Source: CAD feature listing. Evaluate the final solid. Frame: model axes, mm. A direction names the side the tool comes from. Give positions to 0.01 mm unless a question says otherwise; leave off trailing zeros. Loops run counter-clockwise (first coordinate to the right, second up) from the corner with the lowest first, then second, coordinate; pieces in that order, holes last. Notation, with made-up numbers: (18.5, 65.25) -> (40.5, 65.25) arc R21 cw to (40.5, 97.25) -> close; hole circle Ø6 at (32.5, 88). An arc over 180 degrees is marked (long way). Return JSON: item names as keys, results as strings. Group by question number.
Autodesk Inventor part; units mm, degrees
ref_plane "Work Plane1" through (0, 108.1, -624) normal (0, 0, 1) x (1, 0, 0)
ref_plane "YZ Plane" through (0, 0, 0) normal (1, 0, 0) x (0, 1, 0)
ref_plane "XZ Plane" through (0, 0, 0) normal (0, 1, 0) x (-1, 0, 0)
sketch "Sketch1" plane through (0, 0, 0) normal (1, 0, 0) x (0, 1, 0)
  line L0 (107.6, 0) -> (-107.6, 0) construction
  line L1 (108.1, 0) -> (108.1, -40)
  line L2 (108.1, -40) -> (112.1, -40)
  line L3 (112.1, -40) -> (112.1, 12.9)
  line L4 (0, 0) -> (0, 125)
  arc A0 (112.1, 12.9) -> (0, 125) centre (0, 12.9) ccw
  line L5 (108.1, 0) -> (0, 0)
  line L6 (98.1, 0) -> (98.1, 12.9)
  arc A1 (98.1, 12.9) -> (0, 111) centre (0, 12.9) ccw
  line L7 (99.6, 0) -> (99.6, -254) construction
  line L8 (107.6, -254) -> (107.6, 0) construction
  dimension "d0" = 125
  dimension "d2" = 40
  dimension "d5" = 10
  dimension "d8" = 0.5
  dimension "d9" = 4
revolve "Revolution1" add sketch "Sketch1" angle 360 about axis through (0, 0, 0) along (0, 0, 1) contours L5 L6 A1 L4 A0 L3 L2 L1
ref_plane "Work Plane1" through (0, 108.1, -624) normal (0, 0, 1) x (1, 0, 0)
sketch "Sketch6" plane through (0, 0, 0) normal (1, 0, 0) x (0, 1, 0)
  arc A0 (112.1, 12.9) -> (-112.1, 12.9) centre (0, 12.9) ccw construction
  arc A1 (98.1, 12.9) -> (-98.1, 12.9) centre (0, 12.9) ccw construction
  line L0 (98.1, 12.9) -> (98.1, 0) construction
  line L1 (112.1, -40) -> (112.1, 12.9) construction
  line L2 (108.1, 0) -> (108.1, -40) construction
  line L3 (108.1, 0) -> (-108.1, 0) construction
  line L4 (112.1, 12.9) -> (-112.1, 12.9) construction
  arc A2 (108.1, 12.9) -> (0, 121) centre (0, 12.9) ccw
  line L5 (0, 125) -> (132.1, 125)
  line L6 (132.1, 125) -> (132.1, -40)
  line L7 (132.1, -40) -> (108.1, -40)
  line L8 (108.1, 12.9) -> (108.1, -40)
  line L9 (112.1, -40) -> (-112.1, -40)
  line L10 (0, 125) -> (0, 121)
  point P0 (0, 0)
  point P1 (0, 0)
  dimension "d33" = 20
extrude "Extrusion5" add sketch "Sketch6" along normal mid plane 6
sketch "Sketch7" plane through (3, 0, 0) normal (1, 0, 0) x (0, 0, -1)
  arc A0 (-12.9, 112.0599) -> (-124.9599, 0) centre (-12.9, 0) ccw construction
  line L0 (40, 112.0599) -> (-12.9, 112.0599) construction
  line L1 (40, 112.0599) -> (40, 132.1) construction
  line L2 (40, 132.1) -> (-125, 132.1) construction
  line L3 (-125, 132.1) -> (-125, 0) construction
  circle A1 centre (-115, 72.1) radius 5
  circle A2 centre (-115, 97.1) radius 5
  circle A3 centre (-115, 122.1) radius 5
  circle A4 centre (-90, 122.1) radius 5
  circle A5 centre (-65, 122.1) radius 5
  circle A6 centre (-40, 122.1) radius 5
  circle A7 centre (-15, 122.1) radius 5
  circle A8 centre (10, 122.1) radius 5
  circle A9 centre (-90, 97.1) radius 5
  line L4 (-125, 0) -> (-124.9599, 0)
  point P0 (0, 0)
  dimension "d37" = 10
  dimension "d38" = 10
  dimension "d39" = 10
  dimension "d40" = 10
  dimension "d41" = 10
  dimension "d42" = 10
  dimension "d43" = 10
  dimension "d44" = 10
  dimension "d45" = 10
  dimension "d46" = 25
  dimension "d47" = 25
  dimension "d50" = 25
  dimension "d51" = 25
  dimension "d52" = 25
  dimension "d53" = 25
  dimension "d54" = 10
  dimension "d55" = 25
  dimension "d56" = 10
extrude "Extrusion6" cut sketch "Sketch7" against normal through all
fillet "Fillet3" radius 3 4 edges at (3, 66.05, 125) (-3, 66.05, 125) (-3, 132.1, 42.5) (3, 132.1, 42.5)
properties part number "FrontCapV1_3DPrint"
1) Cut plane D-D on x = 0. Count the separate pieces of the cut face and the enclosed holes in it, then the cut area to 3 significant figures.
2) Material intervals for line 1 (Y direction, x = 1, z = 115); line 2 (Y direction, x = 0, z = 115); line 3 (Y direction, x = -1.3, z = 65), sorted ascending.
3) Cut plane B-B on y = 122.1. Return loops of the section in (x, z).
4) Reachability of faces 1 (the face through (0, 65, 125)), 2 (the face through (96, -24, 0)), 3 (the face through (-3, 104, 71)), 4 (the face through (0.042, 126.316, 112.312)) from +Z, -Z, +X, -X, +Y, -Y: full face, straight path, thin tool, end or side. Return the list, or none.
5) Cut plane C-C on z = 90. Return loops of the section in (x, y).
6) Mould query, pull axis Y, two halves, no side actions, for faces 5 (the face through (0, 127, 66)), 6 (the face through (0.1, 132.1, 43.7)), 7 (the face through (3, 104, 71)). Classes: released by +Y, released by -Y, zero draft, split by the parting line, or undercut.
7) Cut plane A-A on z = -10. Return loops of the section in (x, y).
8) Contact query for flat-ended pins moving along their axis: P1, Ø1, axis at x = -55, y = 71.5, coming from the +Z side; P2, Ø8, axis at y = 122.1, z = 40, coming from the -X side; P3, Ø13, axis at y = 122.1, z = 90, coming from the -X side; P4, Ø4, axis at x = 42.5, z = 58, coming from the +Y side. Output: stop coordinate, or through.
Calculated:
{
 "1": {"separate pieces": "1", "enclosed holes": "9", "area": "10,600 mm2"},
 "2": {"line 1": "-46.27 to 67.1, 77.1 to 92.1, 102.1 to 117.1, 127.1 to 131.93", "line 2": "-46.28 to 67.1, 77.1 to 92.1, 102.1 to 117.1, 127.1 to 132.1", "line 3": "-99.25 to -83.11, 83.11 to 117.1, 127.1 to 131.8"},
 "3": {"outline": "(-3, -40) -> (3, -40) -> (3, -15) -> (-3, -15) -> close; (-3, -5) -> (3, -5) -> (3, 10) -> (-3, 10) -> close; (-3, 20) -> (3, 20) -> (3, 35) -> (-3, 35) -> close; (-3, 45) -> (3, 45) -> (3, 60) -> (-3, 60) -> close; (-3, 70) -> (3, 70) -> (3, 85) -> (-3, 85) -> close; (-3, 95) -> (3, 95) -> (3, 110) -> (-3, 110) -> close; (-3, 120) -> (3, 120) -> (3, 122) arc R3 ccw to (-3, 122) -> close"},
 "4": {"face 1": "+Z, +Y", "face 2": "-Z", "face 3": "+Z, -X, +Y", "face 4": "+X, -X"},
 "5": {"outline": "(-3, 81.32) arc R81.38 ccw (long way) to (3, 81.32) -> (3, 92.1) -> (-3, 92.1) -> close; (-3, 102.1) -> (3, 102.1) -> (3, 117.1) -> (-3, 117.1) -> close; (-3, 127.1) -> (3, 127.1) -> (3, 129.1) arc R3 ccw to (-3, 129.1) -> close; hole circle Ø121.31 at (0, 0)"},
 "6": {"face 5": "undercut", "face 6": "released by +Y", "face 7": "zero draft"},
 "7": {"outline": "(-3, 112.06) arc R112.1 ccw (long way) to (3, 112.06) -> (3, 117.1) -> (-3, 117.1) -> close; (-3, 127.1) -> (3, 127.1) -> (3, 129.1) arc R3 ccw to (-3, 129.1) -> close; hole circle Ø216.2 at (0, 0)"},
 "8": {"P1": "z = 80.12", "P2": "through", "P3": "x = -3", "P4": "y = 94.71"}
}
